The listing builds one solid part. Answer for the finished solid, in the listing's coordinates (mm). A direction names the side the tool comes from. Coordinates: 2 decimals unless noted, no trailing zeros. Order: outer loops, then holes, each group sorted by start corner. A loop starts at its lowest first (then second) coordinate and runs counter-clockwise, first axis right, second up. Notation, with made-up numbers: (-20.5, 61) -> (21.5, 61) arc R13 ccw to (21.5, 80) -> close; hole circle Ø9 at (79, -16). An arc over 180 degrees is marked (long way). One line per question, with ' | ' between items.
Autodesk Inventor part; units mm, degrees
ref_plane "Work Plane10" through (-125.6127, 28.0202, 0) normal (0.976, -0.2177, 0) x (0.2177, 0.976, 0)
ref_plane "Work Plane11" through (-125.6127, -28.0202, 0) normal (0.976, 0.2177, 0) x (-0.2177, 0.976, 0)
ref_plane "YZ Plane" through (0, 0, 0) normal (1, 0, 0) x (0, 1, 0)
sketch "Sketch1" plane through (0, 0, 0) normal (0, 0, 1) x (1, 0, 0)
  arc A0 (-113.5134, 34.7045) -> (-113.5134, -34.7045) centre (0, 0) ccw
  line L0 (0, 0) -> (-118.7, 0) construction
  line L1 (0, 0) -> (-113.5134, -34.7045) construction
  line L2 (-113.5134, -34.7045) -> (-113.5134, 0) construction
  line L3 (-113.5134, 0) -> (-113.5134, 34.7045) construction
  arc A1 (-116.3823, 35.5816) -> (-116.3823, -35.5816) centre (0, 0) ccw construction
  line L4 (-113.5134, 34.7045) -> (0, 0) construction
  line L5 (-113.5134, -34.7045) -> (-121.7, -37.2074)
  arc A2 (-113.5134, -34.7045) -> (-113.5134, 34.7045) centre (0, 0) ccw construction
  arc A3 (-116.3823, -35.5816) -> (-116.3823, 35.5816) centre (0, 0) ccw construction
  line L6 (-118.7, 0) -> (-121.7, 0) construction
  line L7 (-121.7, 37.2074) -> (-113.5134, 34.7045)
  line L8 (-121.7, 0) -> (-121.7, 37.2074)
  line L9 (-121.7, 0) -> (-121.7, -37.2074)
  dimension "d0" = 237.4
  dimension "d22" = 17
  dimension "d36" = 3
extrude "Extrusion1" add sketch "Sketch1" along normal mid plane 15
sketch "Sketch11" plane through (0, 0, 0) normal (0, 0, 1) x (1, 0, 0)
  line L0 (-121.7, 37.2074) -> (-121.7, -37.2074)
  line L1 (0, 0) -> (-115.8526, 25.8431) construction
  line L2 (0, 0) -> (-121.7, 0) construction
  line L3 (0, 0) -> (-115.8526, -25.8431) construction
  circle A0 centre (0, 0) radius 124.6911 construction
  arc A1 (-113.5134, 34.7045) -> (-113.5134, -34.7045) centre (0, 0) ccw
  line L4 (-115.8526, 25.8431) -> (-121.7, 27.1474) construction
  line L5 (-115.8526, -25.8431) -> (-121.7, -27.1474) construction
  dimension "d48" = 12.575
  dimension "d49" = 12.575
ref_plane "Work Plane7" through (-115.8526, 25.8431, 0) normal (0.976, -0.2177, 0) x (0.2177, 0.976, 0)
ref_plane "Work Plane8" through (-115.8526, -25.8431, 0) normal (0.976, 0.2177, 0) x (-0.2177, 0.976, 0)
sketch "Sketch12" plane through (-115.8526, 25.8431, 0) normal (0.976, -0.2177, 0) x (0.2177, 0.976, 0)
  line L0 (-4, 0) -> (4, 0) construction
  line L1 (-4, 2.5) -> (4, 2.5)
  line L2 (4, -2.5) -> (-4, -2.5)
  arc A0 (-4, 2.5) -> (-4, -2.5) centre (-4, 0) ccw
  arc A1 (4, -2.5) -> (4, 2.5) centre (4, 0) ccw
  point P0 (0, 0)
  dimension "d50" = 4
  dimension "d51" = 5
extrude "Extrusion10" cut sketch "Sketch12" along normal through all both and the other way through all
sketch "Sketch13" plane through (-115.8526, -25.8431, 0) normal (0.976, 0.2177, 0) x (-0.2177, 0.976, 0)
  line L0 (-4, 0) -> (4, 0) construction
  line L1 (-4, 2.5) -> (4, 2.5)
  line L2 (4, -2.5) -> (-4, -2.5)
  arc A0 (-4, 2.5) -> (-4, -2.5) centre (-4, 0) ccw
  arc A1 (4, -2.5) -> (4, 2.5) centre (4, 0) ccw
  point P0 (0, 0)
  dimension "d54" = 5
  dimension "d55" = 4
extrude "Extrusion11" cut sketch "Sketch13" along normal through all both and the other way through all
ref_plane "Work Plane10" through (-125.6127, 28.0202, 0) normal (0.976, -0.2177, 0) x (0.2177, 0.976, 0)
ref_plane "Work Plane11" through (-125.6127, -28.0202, 0) normal (0.976, 0.2177, 0) x (-0.2177, 0.976, 0)
sketch "Sketch15" plane through (-125.6127, 28.0202, 0) normal (0.976, -0.2177, 0) x (0.2177, 0.976, 0)
  line L0 (5, 0) -> (-5, 0) construction
  line L1 (5, -3.5) -> (-5, -3.5)
  line L2 (-5, 3.5) -> (5, 3.5)
  arc A0 (5, -3.5) -> (5, 3.5) centre (5, 0) ccw
  arc A1 (-5, 3.5) -> (-5, -3.5) centre (-5, 0) ccw
  point P0 (0, 0)
  dimension "d61" = 7
  dimension "d62" = 5
extrude "Extrusion12" [suppressed]
sketch "Sketch16" plane through (-125.6127, -28.0202, 0) normal (0.976, 0.2177, 0) x (-0.2177, 0.976, 0)
  line L0 (5, 0) -> (-5, 0) construction
  line L1 (5, -3.5) -> (-5, -3.5)
  line L2 (-5, 3.5) -> (5, 3.5)
  arc A0 (5, -3.5) -> (5, 3.5) centre (5, 0) ccw
  arc A1 (-5, 3.5) -> (-5, -3.5) centre (-5, 0) ccw
  point P0 (0, 0)
  dimension "d65" = 7
  dimension "d66" = 5
extrude "Extrusion13" [suppressed]
sketch "Sketch19" plane through (0, 0, -7.5) normal (0, 0, -1) x (-1, 0, 0)
  arc A0 (113.5134, -34.7045) -> (113.5134, 34.7045) centre (0, 0) ccw
  arc A1 (111.6008, -34.1198) -> (111.6008, 34.1198) centre (0, 0) ccw
  line L0 (121.7, 37.2074) -> (121.7, -37.2074)
  line L1 (121.7, -37.2074) -> (121.7, 37.2074)
  line L2 (121.7, 37.2074) -> (111.6008, 34.1198)
  line L3 (121.7, -37.2074) -> (111.6008, -34.1198)
  point P0 (0, 0)
  dimension "d75" = 2
extrude "Extrusion15" add sketch "Sketch19" along normal blind 95
sketch "Sketch20" plane through (-121.7, -37.2074, 7.5) normal (-1, 0, 0) x (0, 0, 1)
  line L0 (-107, 3) -> (-18, 3) construction
  line L1 (-18, 3) -> (-18, 71.4148) construction
  line L2 (-18, 71.4148) -> (-107, 71.4148) construction
  line L3 (-107, 71.4148) -> (-107, 3) construction
  line L4 (-15, 2.5029) -> (-15, 71.9119) construction
  line L5 (-110, 74.4148) -> (0, 74.4148)
  line L6 (-110, 0) -> (0, 0)
  line L7 (-110, 0) -> (-110, 74.4148)
  point P0 (-7.5, 37.2074)
  dimension "d78" = 3
  dimension "d79" = 3
  dimension "d80" = 3
  dimension "d81" = 3
  dimension "d82" = 89
  dimension "d83" = 68.4149
hole "Hole1" at (-121.7, 34.2074, -99.5) at (-121.7, 34.2074, -10.5) at (-121.7, -34.2074, -99.5) at (-121.7, -34.2074, -10.5) direction (1, 0, 0) diameter 1 depth 25 tip angle 118
equation "\"d49\" = d48"
equation "\"angulo_alabe\" = 130deg"
equation "\"diametro_tubo\" = 232"
equation "\"desfase_a_pin_superior\" = 12"
equation "\"desfase_b_pin_inferior\" = 8"
equation "\"desfase_b_pin_superior\" = 0"
equation "\"diametro_max_soporte\" = 248"
properties part number "accesorios separador 1"
Item 1: Section A-A, the plane y = 24.5 is taken. Give the vertices of the cut face in (x, z), plus the area to 3 significant figures.
Computed values:
outline: (-121.7, -102.5) -> (-114.1, -102.5) -> (-114.1, -7.5) -> (-116.14, -7.5) -> (-116.14, -2.5) -> (-121.7, -2.5) -> close; (-121.7, 2.5) -> (-116.14, 2.5) -> (-116.14, 7.5) -> (-121.7, 7.5) -> close | area: 778 mm^2
Item 2: Section C-C, the plane y = 1 is taken. Give the vertices of the cut face in (x, z), plus the area to 3 significant figures.
Computed values:
outline: (-121.7, -102.5) -> (-116.7, -102.5) -> (-116.7, -7.5) -> (-118.7, -7.5) -> (-118.7, 7.5) -> (-121.7, 7.5) -> close | area: 520 mm^2
Item 3: For faces 5 (the face through (-116.721, -35.685, -54.335)), 6 (the face through (-119.705, 20.043, -0.055)), 7 (the face through (-118.7, -0.5, -0.1)), 8 (the face through (-118.03, -32.99, -0.05)), 9 (the face through (-116.7, 0.5, -54.3)), determine the directions among +Z, -Z, +X, -X, +Y, -Y from which every point of the face is accessible in a straight line to the end or side of a thin tool.
Computed values:
face 5: +Z, -Z, +X, -Y | face 6: +X | face 7: +Z, +X | face 8: -X | face 9: +Z, -Z, +X
Item 4: Determine the mould class of faces 1 (the face through (-117, 0, -7.5)), 2 (the face through (-118, -26, 2.5)), 3 (the face through (-119.705, -20.043, 0.055)), 4 (the face through (-117.664, 35.973, -0.105)) for opening direction Z: pulls with the +Z half, pulls with the -Z half, needs draft (parallel to the pull), parting line crosses it, or undercut.
Computed values:
face 1: pulls with the +Z half | face 2: undercut | face 3: undercut | face 4: needs draft
Item 5: Each of these flat-tipped pins is pushed along its axis until it touches: pin 1 Ø5 at (y, z) = (14.5, -86.5) entering from +X; pin 2 Ø2 at (x, z) = (-118.5, -19.5) entering from -Y; pin 3 Ø12 at (y, z) = (-3.5, -47) entering from +X. Where does it stop, or does it pass through?
Computed values:
pin 1: stops at x = -115.46 | pin 2: stops at y = -36.53 | pin 3: stops at x = -116.31
Item 6: Find the intervals of material crossed by L1, parallel to Y at x = -117, z = -99.5; L2, parallel to Y at x = -117.5, z = -99.5; L3, parallel to Z at x = -118.25, y = 4, in increasing order.
Computed values:
L1: y = -35.77 to -34.71, -33.71 to 33.71, 34.71 to 35.77 | L2: y = -35.92 to -34.71, -33.71 to 33.71, 34.71 to 35.92 | L3: z = -102.5 to -7.5
Item 7: Section B-B, the plane z = -94.5 is taken. Give the vertices of the cut face in (x, y).
Computed values:
outline: (-121.7, -37.21) -> (-111.6, -34.12) arc R116.7 cw to (-111.6, 34.12) -> (-121.7, 37.21) -> close
